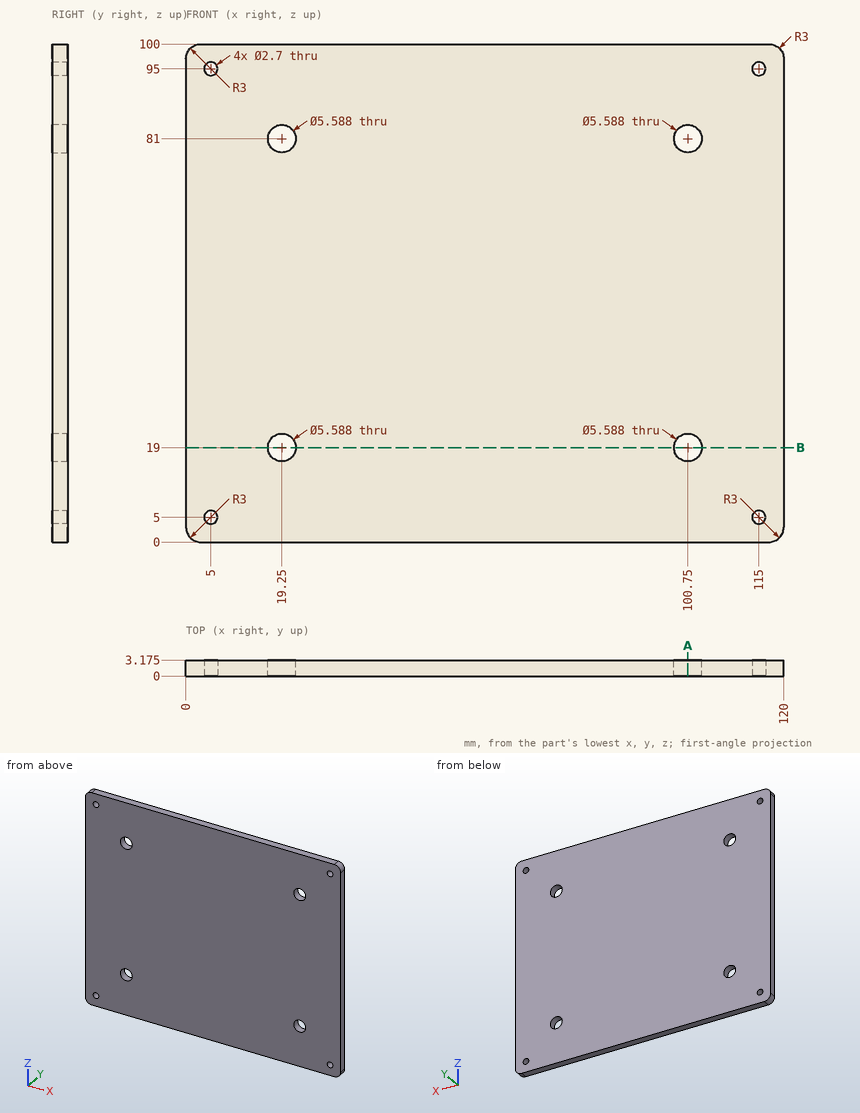
Part print with two shaded views. Sizes in mm from the minimum x, y, z corner. Coordinates: 2 decimals unless noted, no trailing zeros. Order: outer loops, then holes, each group sorted by start corner. A loop starts at its lowest first (then second) coordinate and runs counter-clockwise, first axis right, second up. Notation, with made-up numbers: M 83.25,32.5 L 124.25,32.5 A25 ccw 124.25,64.5 Z; hole C -26,-28.75 d9. An arc over 180 degrees is marked long. Use a Markdown table: item, result.
(1) Cut at B-B on z = 19. Write the cut outline in (x, y) (3 decimals).
A:
| item | result |
|---|---|
| outline | M 0,0 L 16.456,0 L 16.456,3.175 L 0,3.175 Z; M 22.044,0 L 97.956,0 L 97.956,3.175 L 22.044,3.175 Z; M 103.544,0 L 120,0 L 120,3.175 L 103.544,3.175 Z |
(2) Probe L1, parallel to X at y = 1.95, z = 19; L2, parallel to Z at x = 5, y = 1.55; L3, parallel to X at y = 1.05, z = 5. List the from-to ranges inside material, lowest first.
A:
| item | result |
|---|---|
| L1 | x = 0 to 16.46, 22.04 to 97.96, 103.54 to 120 |
| L2 | z = 0 to 3.65, 6.35 to 93.65, 96.35 to 100 |
| L3 | x = 0 to 3.65, 6.35 to 113.65, 116.35 to 120 |
(3) Cut at A-A on x = 100.75. Write the cut outline in (y, z) (3 decimals).
A:
| item | result |
|---|---|
| outline | M 0,0 L 3.175,0 L 3.175,16.206 L 0,16.206 Z; M 0,21.794 L 3.175,21.794 L 3.175,78.206 L 0,78.206 Z; M 0,83.794 L 3.175,83.794 L 3.175,100 L 0,100 Z |
